Verification items for the finished model (mm, model axes). Coordinates: 2 decimals unless noted, no trailing zeros. Order: outer loops, then holes, each group sorted by start corner. A loop starts at its lowest first (then second) coordinate and runs counter-clockwise, first axis right, second up. Notation, with made-up numbers: M 53,-6 L 63,-6 A19 cw 63,4 Z; hole C 43.5,75 d11. An arc over 180 degrees is marked long. Return JSON: item names as keys, results as strings. Group by question number.
1. Section check A-A, the plane y = 1. Give the number of separate pieces and of enclosed holes in the cut face, plus the area to 3 significant figures.
2. Gauge pin test, flat ends, axial feed: pin 1 (6.5 mm diameter, centred on x = 12.1, z = -11.1, fed in from -Y); pin 2 (0.8 mm diameter, centred on x = 11, y = 0.5, fed in from -Z); pin 3 (0.5 mm diameter, centred on x = 11, y = 1, fed in from +Z); pin 4 (0.8 mm diameter, centred on y = 1, z = 13, fed in from -X). Record the tip position at first contact, or that the pin passes through.
3. Section check C-C, the plane x = 2.1. Record the cut outline in (y, z).
4. Section check D-D, the plane x = -4.5. Record the cut outline in (y, z), plus the area to 3 significant figures.
5. Section check B-B, the plane z = -6.4. Record the cut outline in (x, y), plus the area to 3 significant figures.
6. Material ranges on line 1 along X through (y, z) = (0.8, 14); line 2 along Z through (x, y) = (-4.5, 0.55); line 3 along X through (y, z) = (0.75, 14.1), recorded low to high.
7. Mould release check, pull along Y, two halves, no side actions. Record for faces 1 (the flat face through (0, 1.6, 0)), 2 (the flat face through (0, 0, 0)), 3 (the cylindrical face through (-12.374, 0.789, 11.048)): +Y half, -Y half, draft (parallel to the pull), parting line (faces both ways), or undercut.
```python
from build123d import *

# Parameters (mm, degrees)
SKETCH_1_R      = 20.7
SKETCH_1_R_2    = 2
SKETCH_1_R_3    = 1
SKETCH_1_R_4    = 0.363900589
SKETCH_1_R_5    = 0.75
SKETCH_1_W      = 8.030309373
SKETCH_1_H      = 4.588748213
EXTRUDE_1_DEPTH = 1.6


with BuildPart() as part:
    # Эскиз1 → Бобышка-Вытянуть1 (new body)
    with BuildSketch(Plane(origin=(0, 0, 0), x_dir=(1, 0, 0), z_dir=(0, 1, 0))):
        Circle(SKETCH_1_R)
        with Locations((12.1, 11.1)):
            Circle(SKETCH_1_R_2, mode=Mode.SUBTRACT)
        with Locations((-10.9, -12.4)):
            Circle(SKETCH_1_R_2, mode=Mode.SUBTRACT)
        with Locations((-16, 6.4)):
            Circle(SKETCH_1_R_3, mode=Mode.SUBTRACT)
        with Locations((-13.2, 11.3)):
            Circle(SKETCH_1_R_3, mode=Mode.SUBTRACT)
        with Locations((0, 14.5)):
            Circle(SKETCH_1_R_4, mode=Mode.SUBTRACT)
        with Locations((-4.5, 1.6)):
            Circle(SKETCH_1_R_5, mode=Mode.SUBTRACT)
        with Locations((-4.5, -1.6)):
            Circle(SKETCH_1_R_5, mode=Mode.SUBTRACT)
        with Locations((-4.4, -14.1)):
            Circle(SKETCH_1_R_5, mode=Mode.SUBTRACT)
        with Locations((2.1, -14.1)):
            Circle(SKETCH_1_R_5, mode=Mode.SUBTRACT)
        with Locations((9.310736127, -12.60613493)):
            Rectangle(SKETCH_1_W, SKETCH_1_H, mode=Mode.SUBTRACT)
    extrude(amount=EXTRUDE_1_DEPTH)


solid = part.part
```
Answers follow:
{
 "1": {"separate pieces": "1", "enclosed holes": "10", "area": "1,270 mm^2"},
 "2": {"pin 1": "y = 0", "pin 2": "z = -17.78", "pin 3": "z = 17.69", "pin 4": "x = -16.42"},
 "3": {"outline": "M 0,-20.59 L 1.6,-20.59 L 1.6,13.35 L 0,13.35 Z; M 0,14.85 L 1.6,14.85 L 1.6,20.59 L 0,20.59 Z"},
 "4": {"outline": "M 0,-20.2 L 1.6,-20.2 L 1.6,-2.35 L 0,-2.35 Z; M 0,-0.85 L 1.6,-0.85 L 1.6,0.85 L 0,0.85 Z; M 0,2.35 L 1.6,2.35 L 1.6,13.36 L 0,13.36 Z; M 0,14.84 L 1.6,14.84 L 1.6,20.2 L 0,20.2 Z", "area": "57.5 mm^2"},
 "5": {"outline": "M -19.69,0 L -17,0 L -17,1.6 L -19.69,1.6 Z; M -15,0 L 19.69,0 L 19.69,1.6 L -15,1.6 Z", "area": "59.8 mm^2"},
 "6": {"line 1": "-15.25 to -12.1, -9.7 to -5.14, -3.66 to 1.36, 2.84 to 5.3, 13.33 to 15.25", "line 2": "-20.2 to -2.35, -0.85 to 0.85, 2.35 to 13.36, 14.84 to 20.2", "line 3": "-15.16 to -11.95, -9.85 to -5.15, -3.65 to 1.35, 2.85 to 5.3, 13.33 to 15.16"},
 "7": {"face 1": "+Y half", "face 2": "-Y half", "face 3": "draft"}
}
